from build123d import *

# Parameters (mm, degrees)
BOSS_EXTRUDE1_DEPTH            = 1.6
BOSS_EXTRUDE2_DEPTH            = 0.1
M2_HOLE1_FIXINGSTRUCTURE_D     = 2.4
M2_HOLE1_FIXINGSTRUCTURE_DEPTH = 200
M2_HOLE1_FIXINGSTRUCTURE_TIP   = 0.721032743


with BuildPart() as part:
    # Sketch1 → Boss-Extrude1 (new body)
    with BuildSketch(Plane.XY):
        with BuildLine():
            Line((-31.5, 38), (-31.5, 32))
            ThreePointArc((-31.5, 32), (-31.646446609, 31.646446609), (-32, 31.5))
            Line((-32, 31.5), (-38, 31.5))
            ThreePointArc((-38, 31.5), (-38.353553391, 31.353553391), (-38.5, 31))
            Line((-38.5, 31), (-38.5, -31))
            ThreePointArc((-38.5, -31), (-38.353553391, -31.353553391), (-38, -31.5))
            Line((-38, -31.5), (-32, -31.5))
            ThreePointArc((-32, -31.5), (-31.646446609, -31.646446609), (-31.5, -32))
            Line((-31.5, -32), (-31.5, -38))
            ThreePointArc((-31.5, -38), (-31.353553391, -38.353553391), (-31, -38.5))
            Line((-31, -38.5), (31, -38.5))
            ThreePointArc((31, -38.5), (31.353553391, -38.353553391), (31.5, -38))
            Line((31.5, -38), (31.5, -32))
            ThreePointArc((31.5, -32), (31.646446609, -31.646446609), (32, -31.5))
            Line((32, -31.5), (38, -31.5))
            ThreePointArc((38, -31.5), (38.353553391, -31.353553391), (38.5, -31))
            Line((38.5, -31), (38.5, 31))
            ThreePointArc((38.5, 31), (38.353553391, 31.353553391), (38, 31.5))
            Line((38, 31.5), (32, 31.5))
            ThreePointArc((32, 31.5), (31.646446609, 31.646446609), (31.5, 32))
            Line((31.5, 32), (31.5, 38))
            ThreePointArc((31.5, 38), (31.353553391, 38.353553391), (31, 38.5))
            Line((31, 38.5), (-31, 38.5))
            ThreePointArc((-31, 38.5), (-31.353553391, 38.353553391), (-31.5, 38))
        make_face()
    extrude(amount=BOSS_EXTRUDE1_DEPTH)

    # Esboço1 → Boss-Extrude2 (add)
    with BuildSketch(Plane.XY.offset(1.6)):
        with BuildLine():
            Line((-25.5, -36.5), (25.5, -36.5))
            ThreePointArc((25.5, -36.5), (28.721825407, -28.721825407), (36.5, -25.5))
            Line((36.5, -25.5), (36.5, 25.5))
            ThreePointArc((36.5, 25.5), (28.721825407, 28.721825407), (25.5, 36.5))
            Line((25.5, 36.5), (-25.5, 36.5))
            ThreePointArc((-25.5, 36.5), (-28.721825407, 28.721825407), (-36.5, 25.5))
            Line((-36.5, 25.5), (-36.5, -25.5))
            ThreePointArc((-36.5, -25.5), (-28.721825407, -28.721825407), (-25.5, -36.5))
        make_face()
    extrude(amount=BOSS_EXTRUDE2_DEPTH)

    # M2 Hole1-FixingStructure
    with Locations(Plane(origin=(0, 0, 0), x_dir=(-1, 0, 0), z_dir=(0, 0, -1))):
        with Locations((-28, 35), (28, 35), (-28, -35), (28, -35), (35, 28), (35, -28), (-35, -28), (-35, 28)):
            Hole(M2_HOLE1_FIXINGSTRUCTURE_D / 2, depth=M2_HOLE1_FIXINGSTRUCTURE_DEPTH)
            with Locations((0, 0, -(M2_HOLE1_FIXINGSTRUCTURE_DEPTH + M2_HOLE1_FIXINGSTRUCTURE_TIP / 2))):  # 118° drill point
                Cone(0, M2_HOLE1_FIXINGSTRUCTURE_D / 2, M2_HOLE1_FIXINGSTRUCTURE_TIP, mode=Mode.SUBTRACT)


solid = part.part
Could you check a few things on this model? Use its own coordinates, in mm. Give positions to 0.01 mm unless a question says otherwise; leave off trailing zeros. Order: outer loops, then holes, each group sorted by start corner. A loop starts at its lowest first (then second) coordinate and runs counter-clockwise, first axis right, second up.
1. Suppose I cut it at B-B (y = 35). List the corners of the cut face in (x, z) for me, plus the area to 3 significant figures.
2. Suppose I cut it at A-A (z = 0.3). Give the number of separate pieces and of enclosed holes in the cut face, plus the area to 3 significant figures.
3. We'd pull the mould along X, two halves only. Please class faces 1 (the cylindrical face through (-33.89, 27.54, 0.81)), 2 (the flat face through (0, -37, 1.6)), 3 (the cylindrical face through (-27.35, -33.99, 0.81)): pulls with the +X half, pulls with the -X half, needs draft (parallel to the pull), parting line crosses it, or undercut.
4. I need wall thicknesses on L1, parallel to Y at x = -28, z = 1.3; L2, parallel to Y at x = -35, z = 0.9; L3, parallel to Y at x = 33, z = 0.4. Which ranges of each line are inside material? Lowest first, please.
5. Will these pins go through, and if not, where does the flat tip stop? P1, Ø0.5, axis at y = -36.5, z = 0.5, coming from the +X side; P2, Ø1.9, axis at x = -35, y = -28, coming from the -Z side; P3, Ø4, axis at x = -28, y = 35, coming from the -Z side; P4, Ø0.5, axis at x = -35.5, z = 0.5, coming from the +Y side.
Solved:
1. outline: (-31.5, 0) - (-29.2, 0) - (-29.2, 1.6) - (-31.5, 1.6) - close; (-26.8, 0) - (26.8, 0) - (26.8, 1.6) - (25.6, 1.6) - (25.6, 1.7) - (-25.6, 1.7) - (-25.6, 1.6) - (-26.8, 1.6) - close; (29.2, 0) - (31.5, 0) - (31.5, 1.6) - (29.2, 1.6) - close
1. area: 98.2 mm2
2. separate pieces: 1
2. enclosed holes: 8
2. area: 5,700 mm2
3. face 1: undercut
3. face 2: needs draft
3. face 3: undercut
4. L1: y = -38.5 to -36.2, -33.8 to 33.8, 36.2 to 38.5
4. L2: y = -31.5 to -29.2, -26.8 to 26.8, 29.2 to 31.5
4. L3: y = -31.5 to 31.5
5. P1: stops at x = 31.5
5. P2: passes through
5. P3: stops at z = 0
5. P4: stops at y = 31.5
